The listing builds one solid part. Answer for the finished solid, in the listing's coordinates (mm). A direction names the side the tool comes from. Coordinates: 2 decimals unless noted, no trailing zeros. Order: outer loops, then holes, each group sorted by start corner. A loop starts at its lowest first (then second) coordinate and runs counter-clockwise, first axis right, second up. Notation, with made-up numbers: (18, 63.25) -> (55, 63.25) arc R23 cw to (55, 84.25) -> close; hole circle Ø2 at (19, -21). An arc over 180 degrees is marked (long way). Write item = value, one per line.
from build123d import *

# Parameters (mm, degrees)
SKETCH1_R           = 3.175
SKETCH1_R_2         = 1.8161
SKETCH1_R_3         = 7
BOSS_EXTRUDE1_DEPTH = 6.096
SKETCH2_W           = 15.24
SKETCH2_H           = 2.9972
CUT_EXTRUDE1_DEPTH  = 57.86462381
SKETCH3_W           = 2.9972
SKETCH3_H           = 8.89
CUT_EXTRUDE2_DEPTH  = 57.86462381


with BuildPart() as part:
    # Sketch1 → Boss-Extrude1 (new body)
    with BuildSketch(Plane.XY):
        with BuildLine():
            Line((-50.8, 24.815), (50.8, 24.815))
            Line((50.8, 24.815), (50.8, 5.765))
            Line((50.8, 5.765), (12.7, 0))
            ThreePointArc((12.7, 0), (0, -12.7), (-12.7, 0))
            Line((-12.7, 0), (-50.8, 5.765))
            Line((-50.8, 5.765), (-50.8, 24.815))
        make_face()
        with Locations((25.4, 12.7)):
            Circle(SKETCH1_R, mode=Mode.SUBTRACT)
        with Locations((-25.4, 12.7)):
            Circle(SKETCH1_R, mode=Mode.SUBTRACT)
        with Locations((-8.248891971, 4.7625)):
            Circle(SKETCH1_R_2, mode=Mode.SUBTRACT)
        Circle(SKETCH1_R_3, mode=Mode.SUBTRACT)
        with Locations((8.248891971, 4.7625)):
            Circle(SKETCH1_R_2, mode=Mode.SUBTRACT)
        with Locations((0, -9.525)):
            Circle(SKETCH1_R_2, mode=Mode.SUBTRACT)
    extrude(amount=-BOSS_EXTRUDE1_DEPTH)

    # Sketch2 → Cut-Extrude1 (cut, through all)
    with BuildSketch(Plane.XY):
        with Locations((-30.48, 20.7764)):
            Rectangle(SKETCH2_W, SKETCH2_H)
        with Locations((30.48, 20.7764)):
            Rectangle(SKETCH2_W, SKETCH2_H)
    extrude(amount=-CUT_EXTRUDE1_DEPTH, mode=Mode.SUBTRACT)

    # Sketch3 → Cut-Extrude2 (cut, through all)
    with BuildSketch(Plane.XY):
        with Locations((-47.3964, 14.8328)):
            Rectangle(SKETCH3_W, SKETCH3_H)
        with Locations((47.3964, 14.8328)):
            Rectangle(SKETCH3_W, SKETCH3_H)
    extrude(amount=-CUT_EXTRUDE2_DEPTH, mode=Mode.SUBTRACT)


solid = part.part
Q1. The mould has two halves that part along X. Classify faces 1 (the face through (30, 19.278, -3)), 2 (the face through (-1, 24.815, -3)): released by +X, released by -X, zero draft, split by the parting line, or undercut.
The answers:
face_1 = undercut
face_2 = zero draft
Q2. Section A-A, the plane x = 0 is taken. Give the vertices of the cut face in (y, z) (3 decimals), plus the area to 3 significant figures.
The answers:
outline = (-12.7, -6.096) -> (-11.341, -6.096) -> (-11.341, 0) -> (-12.7, 0) -> close; (-7.709, -6.096) -> (-7, -6.096) -> (-7, 0) -> (-7.709, 0) -> close; (7, -6.096) -> (24.815, -6.096) -> (24.815, 0) -> (7, 0) -> close
area = 121 mm2
Q3. Section B-B, the plane y = 12.7 is taken. Give the vertices of the cut face in (x, z) (3 decimals).
The answers:
outline = (-50.8, -6.096) -> (-48.895, -6.096) -> (-48.895, 0) -> (-50.8, 0) -> close; (-45.898, -6.096) -> (-28.575, -6.096) -> (-28.575, 0) -> (-45.898, 0) -> close; (-22.225, -6.096) -> (22.225, -6.096) -> (22.225, 0) -> (-22.225, 0) -> close; (28.575, -6.096) -> (45.898, -6.096) -> (45.898, 0) -> (28.575, 0) -> close; (48.895, -6.096) -> (50.8, -6.096) -> (50.8, 0) -> (48.895, 0) -> close
Q4. Section D-D, the plane z = -1.75 is taken. Give the number of separate pieces and of enclosed holes in the cut face, plus the area to 3 significant figures.
The answers:
separate_pieces = 1
enclosed_holes = 10
area = 2,160 mm2
Q5. Each of these flat-tipped pins is pushed along its axis until it touches: pin 1 Ø5 at (x, y) = (25.4, 12.7) entering from +Z; pin 2 Ø1.8 at (x, z) = (33, -4) entering from -Y; pin 3 Ø1.5 at (x, z) = (-48, -4) entering from -Y; pin 4 Ø3 at (x, z) = (-27, -3.5) entering from -Y. Where does it stop, or does it pass through?
The answers:
pin_1 = through
pin_2 = 2.94
pin_3 = 5.23
pin_4 = 1.94
Q6. Section C-C, the plane y = -5 is taken. Give the vertices of the cut face in (x, z).
The answers:
outline = (-11.67, -6.1) -> (-4.9, -6.1) -> (-4.9, 0) -> (-11.67, 0) -> close; (4.9, -6.1) -> (11.67, -6.1) -> (11.67, 0) -> (4.9, 0) -> close
Q7. A tool of negligible diameter and unlimited length cuts with its end or side. For faces 3 (the face through (1, 15, -6.096)), 4 (the face through (-38.1, 21, -3)), from which of +Z, -Z, +X, -X, +Y, -Y can it reach the whole face along a straight path? Write none if from no direction.
The answers:
face_3 = -Z, +X, -X, +Y, -Y
face_4 = +Z, -Z
Q8. Find the intervals of material crossed by line 1 along Y through (x, z) = (0, -1.25) (3 decimals); line 2 along X through (y, z) = (21.5, -0.5); line 3 along X through (y, z) = (17, -3.75) (3 decimals), in increasing order.
The answers:
line_1 = -12.7 to -11.341, -7.709 to -7, 7 to 24.815
line_2 = -50.8 to -38.1, -22.86 to 22.86, 38.1 to 50.8
line_3 = -50.8 to -48.895, -45.898 to 45.898, 48.895 to 50.8
